The drawing under review shows one solid part. Ordinate dimensions are in mm from its lowest x, y, z. Coordinates: 2 decimals unless noted, no trailing zeros. Order: outer loops, then holes, each group sorted by start corner. A loop starts at its lowest first (then second) coordinate and runs counter-clockwise, first axis right, second up.
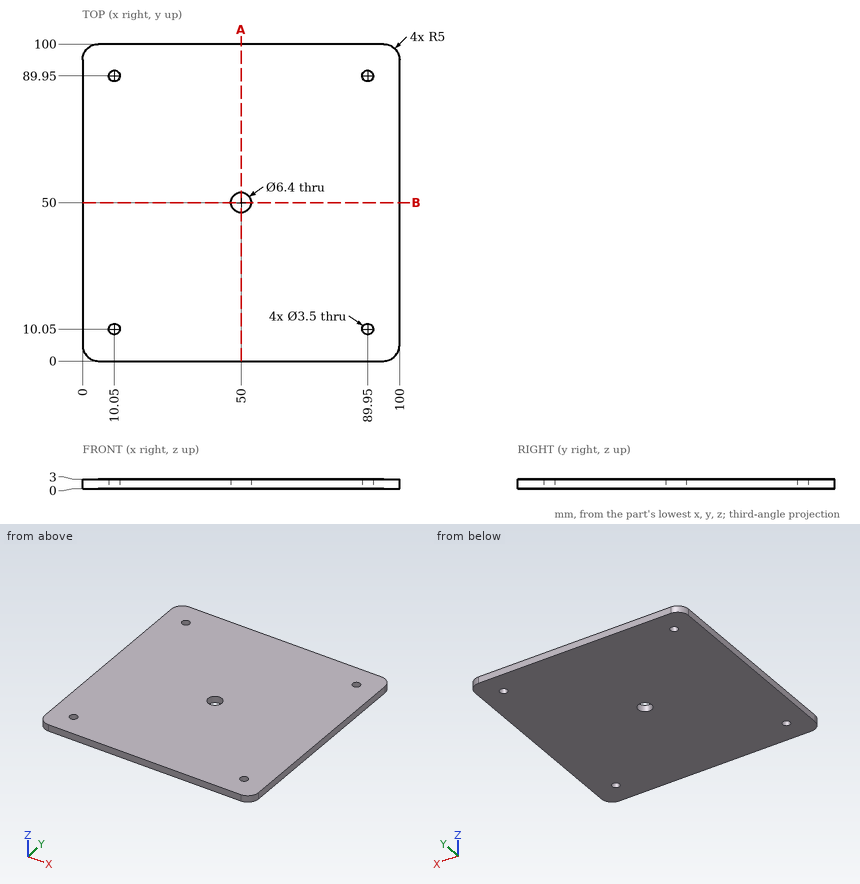
1. Clearance check with a flat-ended pin moving along its axis: pin 1 Ø1 at (y, z) = (72, 2) entering from -X. State where the tip first meets the part, or that it passes through.
Answer below:
pin 1: stops at x = 0
2. Take a section at A-A, the plane x = 50. Give the boundary of the cut face in (y, z), plus the area to 3 significant figures.
Answer below:
outline: (0, 0) - (46.8, 0) - (46.8, 3) - (0, 3) - close; (53.2, 0) - (100, 0) - (100, 3) - (53.2, 3) - close
area: 281 mm2
3. To check wall thickness, follow L1, parallel to Y at x = 50, z = 1.35. State the ranges of the line that lie inside material, in increasing order.
Answer below:
L1: y = 0 to 46.8, 53.2 to 100
